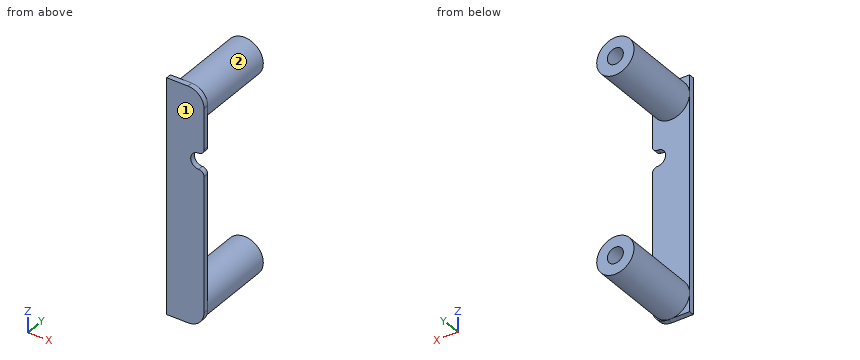
from build123d import *

# Parameters (mm, degrees)
SKETCH1_W               = 44
SKETCH1_H               = 44
BOSS_EXTRUDE1_DEPTH     = 1
SKETCH2_R               = 3.5
BOSS_EXTRUDE2_DEPTH     = 15
SKETCH3_R               = 1.5
CUT_EXTRUDE1_DEPTH      = 15
CUT_EXTRUDE2_DEPTH      = 65.007812023
CUT_EXTRUDE2_DEPTH_BACK = 65.007812023
SKETCH4_W               = 37
SKETCH4_H               = 44
SKETCH5_R               = 1.5
CUT_EXTRUDE3_DEPTH      = 10
FILLET1_R               = 3
FILLET2_R               = 1


with BuildPart() as part:
    # Sketch1 → Boss-Extrude1 (new body)
    with BuildSketch(Plane(origin=(0, 0, 0), x_dir=(1, 0, 0), z_dir=(0, 1, 0))):
        with Locations((22, 22)):
            Rectangle(SKETCH1_W, SKETCH1_H)
    extrude(amount=BOSS_EXTRUDE1_DEPTH)

    # Sketch2 → Boss-Extrude2 (add)
    with BuildSketch(Plane(origin=(0, 1, 0), x_dir=(1, 0, 0), z_dir=(0, 1, 0))):
        with Locations(Location((3.5, 40.5, 0), (0, 0, 90))):
            Circle(SKETCH2_R)
        with Locations(Location((40.5, 40.5, 0), (0, 0, 90))):
            Circle(SKETCH2_R)
        with Locations(Location((40.5, 3.5, 0), (0, 0, 270))):
            Circle(SKETCH2_R)
        with Locations(Location((3.5, 3.5, 0), (0, 0, 270))):
            Circle(SKETCH2_R)
    extrude(amount=BOSS_EXTRUDE2_DEPTH)

    # Sketch3 → Cut-Extrude1 (cut)
    with BuildSketch(Plane(origin=(0, 16, 0), x_dir=(1, 0, 0), z_dir=(0, 1, 0))):
        with Locations(Location((3.5, 40.5, 0), (0, 0, 270))):
            Circle(SKETCH3_R)
        with Locations(Location((40.5, 40.5, 0), (0, 0, 270))):
            Circle(SKETCH3_R)
        with Locations(Location((40.5, 3.5, 0), (0, 0, 270))):
            Circle(SKETCH3_R)
        with Locations(Location((3.5, 3.5, 0), (0, 0, 270))):
            Circle(SKETCH3_R)
    extrude(amount=-CUT_EXTRUDE1_DEPTH, mode=Mode.SUBTRACT)

    # Sketch4 → Cut-Extrude2 (cut, two sides: drawn at the far end of the back side and taken through both)
    with BuildSketch(Plane(origin=(0, 1, 0), x_dir=(1, 0, 0), z_dir=(0, 1, 0)).offset(-CUT_EXTRUDE2_DEPTH_BACK)):
        with Locations((25.5, 22)):
            Rectangle(SKETCH4_W, SKETCH4_H)
    extrude(amount=CUT_EXTRUDE2_DEPTH + CUT_EXTRUDE2_DEPTH_BACK, mode=Mode.SUBTRACT)

    # Sketch5 → Cut-Extrude3 (cut)
    with BuildSketch(Plane(origin=(0, 1, 0), x_dir=(1, 0, 0), z_dir=(0, 1, 0))):
        with Locations((6, 13.2)):
            Circle(SKETCH5_R)
    extrude(amount=-CUT_EXTRUDE3_DEPTH, mode=Mode.SUBTRACT)

    # Fillet1
    fillet1_edges = [part.edges().sort_by_distance(p)[0] for p in [
        (7, 0.5, -44),
        (7, 0.5, 0),
    ]]
    fillet(fillet1_edges, radius=FILLET1_R)

    # Fillet2
    fillet2_edges = [part.edges().sort_by_distance(p)[0] for p in [
        (7, 0.5, -14.318033989),
        (7, 0.5, -12.081966011),
    ]]
    fillet(fillet2_edges, radius=FILLET2_R)


solid = part.part
Can you work these out from the model? Positions are in its coordinate system, mm. Face numbers are marked on the shaded views. Give positions to 0.01 mm unless a question says otherwise; leave off trailing zeros. Write each loop counter-clockwise with the first axis right and the second up, starting at its lowest first coordinate (ties: lowest second). Pieces come first, ordered by that corner, then holes. Notation, with made-up numbers: (9, 66) -> (62, 66) arc R13 cw to (62, 86) -> close; hole circle Ø10 at (20.5, -36). An arc over 180 degrees is marked (long way). Answer as a JSON object with one key per item and string values. Group by question number.
Item 1: We'd pull the mould along Z, two halves only. Please class the marked faces 1 and 2: +Z half, -Z half, draft (parallel to the pull), parting line (faces both ways), or undercut.
Item 2: I'm going to push flat-ended pins straight in: P1, Ø2.5, axis at x = 4, z = -3.5, coming from the +Y side; P2, Ø1, axis at x = 2, y = 8.5, coming from the -Z side; P3, Ø1.5, axis at x = 5, y = 3.5, coming from the +Z side; P4, Ø8, axis at y = 7.5, z = -14.5, coming from the +X side. Where does each tip first touch, or does it pass through?
Item 3: Please list where these lines run through material, in increasing order: line 1 (X direction, y = 8.75, z = -3.5); line 2 (Z direction, x = 4.25, y = 15.25); line 3 (Z direction, x = 4.5, y = 3). Write a range as [from, to].
Item 4: Suppose I cut it at A-A (y = 6.75). Please give me the cut outline in (x, z).
Item 5: Suppose I cut it at C-C (z = -5.5). Please give me the cut outline in (x, y).
Item 6: Suppose I cut it at B-B (z = -13.2). Please give me the cut outline in (x, y), plus the area to 3 significant figures.
Findings:
{
 "1": {"face 1": "draft", "face 2": "undercut"},
 "2": {"P1": "stops at y = 16", "P2": "stops at z = -43.85", "P3": "stops at z = -0.08", "P4": "passes through"},
 "3": {"line 1": "x = [0, 2], [5, 7]", "line 2": "z = [-43.92, -41.8], [-39.2, -37.08], [-6.92, -4.8], [-2.2, -0.08]", "line 3": "z = [-43.85, -41.62], [-39.38, -37.15], [-6.85, -4.62], [-2.38, -0.15]"},
 "4": {"outline": "circle Ø7 at (3.5, -40.5); circle Ø7 at (3.5, -3.5); hole circle Ø3 at (3.5, -40.5); hole circle Ø3 at (3.5, -3.5)"},
 "5": {"outline": "(0, 0) -> (7, 0) -> (7, 1) -> (6.37, 1) -> (6.37, 16) -> (0.63, 16) -> (0.63, 1) -> (0, 1) -> close"},
 "6": {"outline": "(0, 0) -> (4.5, 0) -> (4.5, 1) -> (0, 1) -> close", "area": "4.50 mm²"}
}
